from build123d import *

# Parameters (mm, degrees)
EXTRUDE_THIN1_DEPTH  = 74.25436
FILLET1_RADIUS       = 2.38125
FILLET1_LENGTH       = 74.25436
FILLET2_R            = 2.54
MIRROR1_START        = -74.25436
MIRROR1_DEPTH        = 148.50872
M6_CLEARANCE_HOLE1_D = 6.6
CUT_EXTRUDE5_DEPTH   = 74.25436


# Read off the part's stored shape, not the designer's step: Mirror1
with BuildPart() as part:
    # Sketch4 → Extrude-Thin1 (new body)
    with BuildSketch(Plane.XY):
        Polygon((0, 0), (-50.8, 0), (-50.8, 31.75), (-46.0375, 31.75), (-46.0375, 4.7625), (0, 4.7625), align=None)
    extrude(amount=EXTRUDE_THIN1_DEPTH)

    # Fillet1: full round fillet: the end face becomes a half cylinder, R = half its width
    fillet1_face = Plane((-48.41875, 31.75, 37.12718), x_dir=(0, 0, -1), z_dir=(0, 1, 0))  # on the end face: x along it, z out of the body
    fillet1_slab = fillet1_face.offset(-FILLET1_RADIUS / 2) * Box(FILLET1_LENGTH, 2 * FILLET1_RADIUS, FILLET1_RADIUS, mode=Mode.PRIVATE)  # the body's end, R deep
    fillet1_round = Plane((-48.41875, 29.36875, 37.12718), x_dir=(0, 1, 0), z_dir=(0, 0, -1)) * Cylinder(FILLET1_RADIUS, FILLET1_LENGTH, mode=Mode.PRIVATE)  # its axis R under the face
    add(fillet1_slab - fillet1_round, mode=Mode.SUBTRACT)

    # Fillet2
    fillet2_edges = [part.edges().sort_by_distance(p)[0] for p in [
        (-46.0375, 4.7625, 37.12718),
    ]]
    fillet(fillet2_edges, radius=FILLET2_R)

    # Mirror1 outline → Mirror1 (add)
    with BuildSketch(Plane.XY.offset(MIRROR1_START)):
        with BuildLine():
            ThreePointArc((-46.0375, 29.36875), (-48.41875, 31.75), (-50.8, 29.36875))
            Line((-50.8, 29.36875), (-50.8, 0))
            Line((-50.8, 0), (50.8, 0))
            Line((50.8, 0), (50.8, 29.36875))
            ThreePointArc((50.8, 29.36875), (48.41875, 31.75), (46.0375, 29.36875))
            Line((46.0375, 29.36875), (46.0375, 7.3025))
            ThreePointArc((46.0375, 7.3025), (45.293551224, 5.506448776), (43.4975, 4.7625))
            Line((43.4975, 4.7625), (-43.4975, 4.7625))
            ThreePointArc((-43.4975, 4.7625), (-45.293551224, 5.506448776), (-46.0375, 7.3025))
            Line((-46.0375, 7.3025), (-46.0375, 29.36875))
        make_face()
    extrude(amount=MIRROR1_DEPTH)

    # M6 Clearance Hole1 (through all)
    with Locations(Plane(origin=(-33.02, 0, 61.87186), x_dir=(0, 0, -1), z_dir=(0, -1, 0))):
        with Locations((0, 0), (0, 66.04), (123.74372, 0), (123.74372, 66.04)):
            Hole(M6_CLEARANCE_HOLE1_D / 2)

    # Sketch12 → Cut-Extrude5 (cut, symmetric)
    with BuildSketch(Plane.XY):
        Polygon((-50.8, 0.254), (50.8, 0.254), (50.8, 0), (50.8, -4.927247647), (-50.8, -4.927247647), (-50.8, 0), align=None)
    extrude(amount=CUT_EXTRUDE5_DEPTH, both=True, mode=Mode.SUBTRACT)


solid = part.part
Verification items for the finished model (mm, model axes). A direction names the side the tool comes from. Coordinates: 2 decimals unless noted, no trailing zeros. Write each loop counter-clockwise with the first axis right and the second up, starting at its lowest first coordinate (ties: lowest second). Pieces come first, ordered by that corner, then holes. Notation, with made-up numbers: (-6, 23.5) - (15, 23.5) arc R9 ccw to (15, 29.5) - close; hole circle Ø6 at (28, 53.5). An arc over 180 degrees is marked (long way). Answer as a JSON object with one key per item and string values.
(1) Tool access check on faces 4 (the flat face through (-46.038, 18, -1)), 5 (the cylindrical face through (-30.79, 2.54, 59.44)). Record the directions out of +Z, -Z, +X, -X, +Y, -Y that give a thin tool (end or side, any length) a straight path to the whole face; none if there is none.
Report:
{"face 4": "+Z, -Z, +Y", "face 5": "+Y, -Y"}
(2) Mould release check, pull along X, two halves, no side actions. Record for faces 1 (the cylindrical face through (-32.029, 2.54, -58.724)), 2 (the flat face through (0, 4, 74.254)), 3 (the flat face through (-50.8, 15, -1)): pulls with the +X half, pulls with the -X half, needs draft (parallel to the pull), parting line crosses it, or undercut.
Report:
{"face 1": "undercut", "face 2": "needs draft", "face 3": "pulls with the -X half"}
(3) Cross-section at C-C on z = -63. Record the cut outline in (x, y).
Report:
{"outline": "(-50.8, 0.25) - (-36.12, 0.25) - (-36.12, 4.76) - (-43.5, 4.76) arc R2.54 cw to (-46.04, 7.3) - (-46.04, 29.37) arc R2.38 ccw to (-50.8, 29.37) - close; (-29.92, 0.25) - (29.92, 0.25) - (29.92, 4.76) - (-29.92, 4.76) - close; (36.12, 0.25) - (50.8, 0.25) - (50.8, 29.37) arc R2.38 ccw to (46.04, 29.37) - (46.04, 7.3) arc R2.54 cw to (43.5, 4.76) - (36.12, 4.76) - close"}
(4) Cross-section at D-D on z = 2. Record the cut outline in (x, y).
Report:
{"outline": "(-50.8, 0.25) - (50.8, 0.25) - (50.8, 29.37) arc R2.38 ccw to (46.04, 29.37) - (46.04, 7.3) arc R2.54 cw to (43.5, 4.76) - (-43.5, 4.76) arc R2.54 cw to (-46.04, 7.3) - (-46.04, 29.37) arc R2.38 ccw to (-50.8, 29.37) - close"}
(5) Gauge pin test, flat end, axial feed: pin 1 Ø3 at (x, z) = (33, 8) entering from +Y. Record the tip position at first contact, or that the pin passes through.
Report:
{"pin 1": "y = 4.76"}
(6) Cross-section at B-B on x = 33.02. Record the cut outline in (y, z), plus the area to 3 significant figures.
Report:
{"outline": "(0.25, -74.25) - (4.76, -74.25) - (4.76, -65.17) - (0.25, -65.17) - close; (0.25, -58.57) - (4.76, -58.57) - (4.76, 58.57) - (0.25, 58.57) - close; (0.25, 65.17) - (4.76, 65.17) - (4.76, 74.25) - (0.25, 74.25) - close", "area": "610 mm^2"}
(7) Cross-section at A-A on y = 16. Record the cut outline in (x, z).
Report:
{"outline": "(-50.8, -74.25) - (-46.04, -74.25) - (-46.04, 74.25) - (-50.8, 74.25) - close; (46.04, -74.25) - (50.8, -74.25) - (50.8, 74.25) - (46.04, 74.25) - close"}
(8) Thickness scan on line 1 along X through (y, z) = (25.5, 37.5); line 2 along Y through (x, z) = (-35, 34); line 3 along X through (y, z) = (5.5, 11). Record the ranges inside material, lowest first.
Report:
{"line 1": "-50.8 to -46.04, 46.04 to 50.8", "line 2": "0.25 to 4.76", "line 3": "-50.8 to -45.29, 45.29 to 50.8"}
